```python
from build123d import *

# Parameters (mm, degrees)
BOSS_EXTRUDE1_DEPTH = 2.54
FILLET1_R           = 2.54


with BuildPart() as part:
    # Sketch1 → Boss-Extrude1 (new body)
    with BuildSketch(Plane(origin=(0, 0, 0), x_dir=(0, 0, -1), z_dir=(1, 0, 0))):
        with BuildLine():
            ThreePointArc((-57.404, 88.9), (-53.848, 92.456), (-50.292, 88.9))
            Line((-50.292, 88.9), (-44.45, 82.55))
            Line((-44.45, 82.55), (-38.608, 88.9))
            ThreePointArc((-38.608, 88.9), (-35.052, 92.456), (-31.496, 88.9))
            Line((-31.496, 88.9), (-25.4, 82.55))
            Line((-25.4, 82.55), (-25.4, 0))
            Line((-25.4, 0), (0, 0))
            Line((0, 0), (52.41925, 32.385))
            Line((52.41925, 32.385), (52.41925, 40.64))
            Line((52.41925, 40.64), (9.734598471, 101.6))
            ThreePointArc((9.734598471, 101.6), (-33.232700765, 123.967360233), (-76.2, 101.6))
            Line((-76.2, 101.6), (-76.2, 69.320833333))
            Line((-76.2, 69.320833333), (-57.404, 88.9))
        make_face()
    extrude(amount=BOSS_EXTRUDE1_DEPTH)

    # Fillet1
    fillet1_edges = [part.edges().sort_by_distance(p)[0] for p in [
        (1.27, 40.64, -52.41925),
        (1.27, 32.385, -52.41925),
        (1.27, 0, 0),
        (1.27, 0, 25.4),
        (1.27, 82.55, 25.4),
        (1.27, 88.9, 31.496),
        (1.27, 88.9, 38.608),
        (1.27, 82.55, 44.45),
        (1.27, 88.9, 50.292),
        (1.27, 88.9, 57.404),
        (1.27, 69.320833333, 76.2),
        (1.27, 101.6, 76.2),
    ]]
    fillet(fillet1_edges, radius=FILLET1_R)


solid = part.part
```
The listing builds one solid part. Answer for the finished solid, in the listing's coordinates (mm). A direction names the side the tool comes from. Round coordinates to 2 decimals unless told otherwise and drop trailing zeros. Write each loop counter-clockwise with the first axis right and the second up, starting at its lowest first coordinate (ties: lowest second). Pieces come first, ordered by that corner, then holes. Notation, with made-up numbers: (7, -8) -> (29, -8) arc R15 cw to (29, 4) -> close; hole circle Ø4 at (-24.75, -40). An arc over 180 degrees is marked (long way). Answer as a JSON object with one key per item and string values. Group by question number.
Q1. Section B-B (y = 62) is taken. Write down the section's boundary in (x, z).
Q2. Section C-C (z = -12) is taken. Write down the section's boundary in (x, y), plus the area to 3 significant figures.
Q3. Determine the mould class of faces 1 (the face through (1.252, 86.405, 40.904)), 2 (the face through (1.252, 123.956, 32.118)), 3 (the face through (2.54, 63, 13)) for opening direction Z: pulls with the +Z half, pulls with the -Z half, needs draft (parallel to the pull), parting line crosses it, or undercut.
Q4. Straight lines are drawn through the part: line 1 along Z through (x, y) = (1.65, 90); line 2 along Z through (x, y) = (2.35, 80); line 3 along Z through (x, y) = (1.15, 74.5). For each, find the intervals that lie inside material, in ascending order.
Q5. Which of the six approach directions +Z, -Z, +X, -X, +Y, -Y give full straight-line access (tool end or side, diameter ignored) to faces 4 (the face through (1.25, 71.03, -31.14)), 5 (the face through (1.252, 85.815, 28.535))?
Q6. Section A-A (x = 1.2) is taken. Write down the section's boundary in (y, z), plus the area to 3 significant figures.
Q7. This flat-tipped pin is pushed along its axis until it touches: pin 1 Ø1.5 at (x, y) = (1, 80.5) entering from -Z. Where does it stop, or does it pass through?
Check values:
{
 "1": {"outline": "(0, -37.46) -> (2.54, -37.46) -> (2.54, 25.4) -> (0, 25.4) -> close"},
 "2": {"outline": "(0, 7.41) -> (2.54, 7.41) -> (2.54, 98.36) -> (0, 98.36) -> close", "area": "231 mm^2"},
 "3": {"face 1": "undercut", "face 2": "parting line crosses it", "face 3": "needs draft"},
 "4": {"line 1": "-17.86 to 31.67, 38.43 to 50.47, 57.23 to 76.2", "line 2": "-24.86 to 25.4, 65.95 to 76.2", "line 3": "-28.71 to 25.4, 71.23 to 75.93"},
 "5": {"face 4": "-Z, +X, -X, +Y", "face 5": "+X, -X, -Y"},
 "6": {"outline": "(0, 0.72) arc R2.54 ccw to (0.38, -0.61) -> (31.64, -51.21) arc R2.54 ccw to (33.8, -52.42) -> (39.84, -52.42) arc R2.54 ccw to (41.3, -51.96) -> (101.6, -9.73) arc R52.45 ccw to (102.28, 75.72) arc R2.54 ccw to (100.79, 76.2) -> (75.63, 76.2) arc R2.54 ccw to (73.88, 71.83) -> (88.27, 58.01) arc R2.54 ccw to (89.56, 57.34) arc R3.56 cw to (89.54, 50.35) arc R2.54 ccw to (88.28, 49.72) -> (84.58, 46.32) arc R2.54 ccw to (84.58, 42.58) -> (88.28, 39.18) arc R2.54 ccw to (89.54, 38.55) arc R3.56 cw to (89.56, 31.56) arc R2.54 ccw to (88.27, 30.89) -> (83.29, 26.11) arc R2.54 cw to (81.53, 25.4) -> (2.54, 25.4) arc R2.54 ccw to (0, 22.86) -> close", "area": "7,940 mm^2"},
 "7": {"pin 1": "z = -25.03"}
}
